Solid Edge part; units mm, degrees
sketch "Sketch1" plane through (0, 0, 0) normal (0, 0, 1) x (1, 0, 0)
  circle A0 centre (0, 0) radius 42.5325
extrude "Protrusion1" add sketch "Sketch1" along normal blind 111.0642
sketch "Sketch2" plane through (0, 0, 0) normal (1, 0, 0) x (0, 1, 0)
  line L0 (-34.4095, 0) -> (0, 26.2845)
extrude "ExtrudedCutout_6" cut sketch "Sketch2" along normal mid plane 236.5553 material side at (0, -17.2351, 13.182)
pattern_circular "Pattern1" count 5 over 360 about axis through (0, 0, 0) along (0, 0, 1) of "ExtrudedCutout_6"
sketch "Sketch3" plane through (0, 0, 0) normal (0, 0, 1) x (1, 0, 0)
  circle A0 centre (0, 0) radius 42.5325
extrude "ExtrudedProtrusion_3" add sketch "Sketch3" against normal blind 146.9962
sketch "Sketch4" plane through (0, 0, 0) normal (1, 0, 0) x (0, 1, 0)
  line L0 (-34.4095, 0) -> (-42.5325, -42.5312)
extrude "ExtrudedCutout_11" cut sketch "Sketch4" along normal mid plane 186.9173 material side at (0, -38.5201, -21.2562)
pattern_circular "Pattern2" count 5 over 360 about axis through (0, 0, 0) along (0, 0, 1) of "ExtrudedCutout_11"
sketch "Sketch5" plane through (0, 0, -146.9962) normal (0, 0, -1) x (0, 1, 0)
  circle A0 centre (0, 0) radius 42.5325
extrude "Cutout9" cut sketch "Sketch5" along normal mid plane 208.93
sketch "Sketch6" plane through (0, 0, 0) normal (1, 0, 0) x (0, 1, 0)
  line L0 (34.4237, -42.5312) -> (42.5325, 0)
extrude "ExtrudedCutout_19" cut sketch "Sketch6" along normal mid plane 152.0733 material side at (0, 38.5272, -21.275)
pattern_circular "Pattern3" count 5 over 360 about axis through (0, 0, -42.5312) along (0, 0, -1) of "ExtrudedCutout_19"
sketch "Sketch7" plane through (0, -4.0567, -42.5312) normal (0, 0, -1) x (1, 0, 0)
  line L0 (-25, -38.4662) -> (25, -38.4662)
  line L1 (25, -38.4662) -> (40.4509, 9.0866)
  line L2 (40.4509, 9.0866) -> (0, 38.4758)
  line L3 (0, 38.4758) -> (-40.4508, 9.0866)
  line L4 (-40.4508, 9.0866) -> (-25, -38.4662)
extrude "ExtrudedProtrusion_5" add sketch "Sketch7" along normal blind 53.0273
sketch "Sketch8" plane through (0, 0, 0) normal (1, 0, 0) x (0, 1, 0)
  line L0 (34.4095, -42.5312) -> (0, -68.8157)
extrude "ExtrudedCutout_29" cut sketch "Sketch8" along normal mid plane 468.9384 material side at (0, 17.2351, -55.7132)
pattern_circular "Pattern4" count 5 over 360 about axis through (0, 0, 0) along (0, 0, 1) of "ExtrudedCutout_29"
Work out the finished part from the listing and answer in its coordinate system (mm). Round coordinates to 2 decimals unless told otherwise and drop trailing zeros. Order: outer loops, then holes, each group sorted by start corner. A loop starts at its lowest first (then second) coordinate and runs counter-clockwise, first axis right, second up.
Q1. A cutting plane is placed at C-C, the plane y = -28. Determine the outline of the cut face in (x, z).
Solution:
outline: (-29.66, -12.83) - (-20.03, -42.52) - (0, -51.51) - (20.03, -42.52) - (29.66, -12.83) - (27.08, 0) - (20.34, 4.9) - (-20.34, 4.9) - (-27.08, 0) - close
Q2. A cutting plane is placed at A-A, the plane x = -2.5. Determine the outline of the cut face in (y, z).
Solution:
outline: (-41.73, -38.32) - (-40.74, -42.52) - (-0.81, -67.19) - (3.44, -66.19) - (34.43, -42.52) - (41.72, -4.26) - (40.72, 0) - (0.81, 24.66) - (-3.44, 23.66) - (-34.41, 0) - close
Q3. A cutting plane is placed at D-D, the plane x = -18.5. Determine the outline of the cut face in (y, z), then the cut area to 3 significant figures.
Solution:
outline: (-36.52, -11.07) - (-29.11, -42.52) - (-6.01, -56.79) - (25.46, -49.37) - (34.43, -42.52) - (36.53, -31.5) - (29.09, 0) - (6.01, 14.26) - (-25.46, 6.83) - (-34.41, 0) - close
area: 3,900 mm2
Q4. Given pin 1 Ø1 at (x, y) = (-23.5, 20) entering from +Z; pin 2 Ø1.5 at (x, y) = (19, 24) entering from +Z; pin 3 Ø5 at (y, z) = (-3.5, -34) entering from -X, each flat-ended and moving along its own axis, determine where each tip first touches the part or whether it passes through.
Solution:
pin 1: stops at z = 3.76
pin 2: stops at z = 3.49
pin 3: stops at x = -40
Q5. A cutting plane is placed at B-B, the plane z = 5.5. Determine the outline of the cut face in (x, y), then the cut area to 3 significant figures.
Solution:
outline: (-31.99, 10.39) - (-19.77, -27.21) - (19.77, -27.21) - (31.99, 10.39) - (0, 33.63) - close
area: 2,690 mm2
Q6. Find the intervals of material crossed by line 1 along Z through (x, y) = (-13.5, -1); line 2 along X through (y, z) = (-2, -42.5); line 3 along Z through (x, y) = (-8, 13), in increasing order.
Solution:
line 1: z = -59.24 to 16.24
line 2: x = -36.85 to 36.85
line 3: z = -58.89 to 14.66
